Here's how the part is built. I have some questions about the finished solid (model axes, mm). A direction names the side the tool comes from. Round coordinates to 2 decimals unless told otherwise and drop trailing zeros. Loops run counter-clockwise (first coordinate to the right, second up) from the corner with the lowest first, then second, coordinate; pieces in that order, holes last. Notation, with made-up numbers: (-23.5, -18.5) -> (22.5, -18.5) arc R25 ccw to (22.5, 13.5) -> close; hole circle Ø7 at (-32, 28.5). An arc over 180 degrees is marked (long way). One line per item, written item: value. Start each with the question number.
```python
from build123d import *

# Parameters (mm, degrees)
F0_W     = 51.813559141
F0_H     = 32.5880763121
F1_DEPTH = 25.4
F2_DEPTH = 25.4
F3_DEPTH = 25.4
F4_DEPTH = 7.1882
F6_DEPTH = 37.846
F7_R     = 6.35
F8_DEPTH = 50.8
F9_DEPTH = 4.572


# Not quite as in the source:
# - a feature of the source that left no trace in its solid (it failed there, or was rolled back) is left out


with BuildPart() as f1:
    # F0 (on Front) → F1 (new body)
    with BuildSketch(Plane.XZ):
        with Locations((-23.6830220092, 10.7818876859)):
            Rectangle(F0_W, F0_H)
    extrude(amount=F1_DEPTH)

    # F2 (add): a face of the model
    f2_faces = [f1.faces().sort_by_distance(p)[0] for p in [
        (-23.6830220092, -25.4, 10.7818876859),
    ]]
    extrude(f2_faces, amount=F2_DEPTH)

    # F3 (add): a face of the model
    f3_faces = [f1.faces().sort_by_distance(p)[0] for p in [
        (-23.6830220092, -25.4, 27.0759258419),
    ]]
    extrude(f3_faces, amount=F3_DEPTH)

    # F4 (add): a face of the model
    f4_faces = [f1.faces().sort_by_distance(p)[0] for p in [
        (-23.6830220092, -25.4, 52.4759258419),
    ]]
    extrude(f4_faces, amount=-F4_DEPTH)

    # F5 (on face) → F6 (cut)
    with BuildSketch(Plane.XY.offset(52.4759258419)):
        Polygon((-36.8200466037, 0), (-36.8200466037, -25.4), (-36.8200466037, -50.8), (2.2237575613, -50.8), (2.2237575613, 0), align=None)
    extrude(amount=-F6_DEPTH, mode=Mode.SUBTRACT)

    # F7 (on face) → F8 (cut)
    with BuildSketch(Plane.YZ.offset(-36.8200466037)):
        with Locations((-24.1173226386, 35.6486514211)):
            Circle(F7_R)
    extrude(amount=-F8_DEPTH, mode=Mode.SUBTRACT)

    # F9 (cut): a face of the model
    f9_faces = [f1.faces().sort_by_distance(p)[0] for p in [
        (-17.2981445212, -25.4, 14.6299258419),
    ]]
    extrude(f9_faces, amount=-F9_DEPTH, mode=Mode.SUBTRACT)


solid = f1.part
```
Q1. If I drill on line 1 along X through (y, z) = (-4.5, 24); line 2 along Z through (x, y) = (-18, -6.5); line 3 along Z through (x, y) = (-45, -23.5), over which ranges is the centre line in solid material (lowest first)?
Q2. I want a section at D-D on y = -10.5. Please give me the cut outline in (x, z).
Q3. I want a section at C-C on z = 21. Please give me the cut outline in (x, y).
Q4. Will these pins go through, and if not, where does the flat tip stop? P1, Ø10, axis at x = -13, z = 10, coming from the +Y side; P2, Ø19.5, axis at x = -20.5, y = -13.5, coming from the +Z side; P3, Ø3, axis at y = -41, z = 29, coming from the +X side.
Q5. I want a section at B-B on x = -42. Please give me the cut outline in (y, z).
Q6. I want a section at A-A on y = -21.5. Please give me the cut outline in (x, z).
Q7. If we mould it in two halves opening along Y, with no side actions, what happens to faces 1 (the flat face through (-41, -50.8, 11)), 2 (the cylindrical face through (-43.12, -25.49, 29.45)), 3 (the flat face through (-43, -25, 52.476))? For each: released by +Y, released by -Y, zero draft, split by the parting line, or undercut.
Q8. Which directions (+Z, -Z, +X, -X, +Y, -Y) give clear straight access to the entire face, cutting with the end or side of a thin tool? Please do faces 4 (the flat face through (-36.82, -25, 27)), 5 (the flat face through (-49.59, -26, 24)).
Answers below:
1. line 1: x = -49.59 to -36.82
1. line 2: z = -5.51 to 10.06
1. line 3: z = -5.51 to 29.33, 41.97 to 52.48
2. outline: (-49.59, -5.51) -> (2.22, -5.51) -> (2.22, 10.06) -> (-36.82, 10.06) -> (-36.82, 52.48) -> (-49.59, 52.48) -> close
3. outline: (-49.59, -50.8) -> (-36.82, -50.8) -> (-36.82, 0) -> (-49.59, 0) -> close
4. P1: stops at y = 0
4. P2: stops at z = 10.06
4. P3: stops at x = -36.82
5. outline: (-50.8, -5.51) -> (0, -5.51) -> (0, 52.48) -> (-50.8, 52.48) -> close; hole circle Ø12.7 at (-24.12, 35.65)
6. outline: (-49.59, -5.51) -> (2.22, -5.51) -> (2.22, 10.06) -> (-36.82, 10.06) -> (-36.82, 29.86) -> (-49.59, 29.86) -> close; (-49.59, 41.43) -> (-36.82, 41.43) -> (-36.82, 52.48) -> (-49.59, 52.48) -> close
7. face 1: released by -Y
7. face 2: undercut
7. face 3: zero draft
8. face 4: +Z, +X, +Y, -Y
8. face 5: +Z, -Z, -X, +Y, -Y
